```python
from build123d import *

# Parameters (mm, degrees)
SKETCH1_W           = 6.35
SKETCH1_H           = 20.32
SKETCH1_R           = 2.032
BOSS_EXTRUDE1_DEPTH = 11.43
SKETCH1_3_R         = 2.032
CUT_EXTRUDE1_DEPTH  = 6.35
SKETCH2_R           = 2.032
CUT_EXTRUDE2_DEPTH  = 17.558774109
CHAMFER1_SIZE       = 6.35
FILLET1_R           = 6.35
FILLET2_R           = 6.35
CHAMFER2_SIZE       = 0.635
CHAMFER3_SIZE       = 0.635


with BuildPart() as part:
    # Sketch1 → Boss-Extrude1 (new body)
    # profile 1 of 3: a face of its own
    with BuildSketch(Plane(origin=(0, 0, 0), x_dir=(1, 0, 0), z_dir=(0, 1, 0))):
        Rectangle(SKETCH1_W, SKETCH1_H)
        with Locations((0, -6.35)):
            Circle(SKETCH1_R, mode=Mode.SUBTRACT)
        with Locations((0, 6.35)):
            Circle(SKETCH1_R, mode=Mode.SUBTRACT)
    # profile 2 of 3: a face of its own
    with BuildSketch(Plane(origin=(0, 0, 0), x_dir=(1, 0, 0), z_dir=(0, 1, 0))):
        with Locations((0, -6.35)):
            Circle(SKETCH1_R)
    # profile 3 of 3: a face of its own
    with BuildSketch(Plane(origin=(0, 0, 0), x_dir=(1, 0, 0), z_dir=(0, 1, 0))):
        with Locations((0, 6.35)):
            Circle(SKETCH1_R)
    extrude(amount=BOSS_EXTRUDE1_DEPTH)

    # Sketch1<3> → Cut-Extrude1 (cut)
    with BuildSketch(Plane(origin=(0, 0, 0), x_dir=(1, 0, 0), z_dir=(0, 1, 0))):
        with Locations(Location((0, 6.35, 0), (0, 0, 270))):
            Circle(SKETCH1_3_R)
        with Locations(Location((0, -6.35, 0), (0, 0, 270))):
            Circle(SKETCH1_3_R)
    extrude(amount=CUT_EXTRUDE1_DEPTH, mode=Mode.SUBTRACT)

    # Sketch2 → Cut-Extrude2 (cut, through all)
    with BuildSketch(Plane(origin=(3.175, 0, 0), x_dir=(0, 0, -1), z_dir=(1, 0, 0))):
        with Locations((0, 7.62)):
            Circle(SKETCH2_R)
    extrude(amount=-CUT_EXTRUDE2_DEPTH, mode=Mode.SUBTRACT)

    # Chamfer1
    chamfer1_edges = [part.edges().sort_by_distance(p)[0] for p in [
        (0, 11.43, -10.16),
        (0, 11.43, 10.16),
    ]]
    chamfer(chamfer1_edges, length=CHAMFER1_SIZE)

    # Fillet1
    fillet1_edges = [part.edges().sort_by_distance(p)[0] for p in [
        (0, 11.43, 3.81),
        (0, 11.43, -3.81),
    ]]
    fillet(fillet1_edges, radius=FILLET1_R)

    # Fillet2
    fillet2_edges = [part.edges().sort_by_distance(p)[0] for p in [
        (0, 5.08, -10.16),
        (0, 5.08, 10.16),
    ]]
    fillet(fillet2_edges, radius=FILLET2_R)

    # Chamfer2
    chamfer2_edges = [part.edges().sort_by_distance(p)[0] for p in [
        (3.175, 11.43, 0),
        (-3.175, 11.43, 0),
        (-3.175, 8.255, -6.985),
        (-3.175, 10.946635031, 3.609783674),
        (-3.175, 10.946635031, -3.609783674),
        (3.175, 8.255, 6.985),
        (3.175, 10.946635031, 3.609783674),
        (3.175, 10.946635031, -3.609783674),
        (-3.175, 0, 0),
        (-3.175, 1.224871939, -10.16),
        (3.175, 1.224871939, -10.16),
        (3.175, 8.255, -6.985),
        (3.175, 1.224871939, 10.16),
        (3.175, 4.879783674, 9.676635031),
        (3.175, 4.879783674, -9.676635031),
        (-3.175, 1.224871939, 10.16),
        (0, 0, -10.16),
        (-3.175, 8.255, 6.985),
        (-3.175, 4.879783674, 9.676635031),
        (-3.175, 4.879783674, -9.676635031),
        (3.175, 0, 0),
        (0, 0, 10.16),
    ]]
    chamfer(chamfer2_edges, length=CHAMFER2_SIZE)

    # Chamfer3
    # the kernel refuses this chamfer: 0.635 mm, written as the material it takes off along each edge
    with BuildSketch(Plane(origin=(0, 0, 6.35), x_dir=(0, 0, 1), z_dir=(-1, 0, 0))) as chamfer3_piece_1:
        Polygon((2.032 + CHAMFER3_SIZE, 0), (2.032, CHAMFER3_SIZE), (2.032, 0), align=None)
    revolve(axis=Axis((0, 0, 6.35), (0, 1, 0)), mode=Mode.SUBTRACT)
    with BuildSketch(Plane(origin=(0, 0, -6.35), x_dir=(0, 0, 1), z_dir=(-1, 0, 0))) as chamfer3_piece_2:
        Polygon((2.032 + CHAMFER3_SIZE, 0), (2.032, CHAMFER3_SIZE), (2.032, 0), align=None)
    revolve(axis=Axis((0, 0, -6.35), (0, 1, 0)), mode=Mode.SUBTRACT)
    with BuildSketch(Plane(origin=(-3.175, 7.62, 0), x_dir=(0, 0, -1), z_dir=(0, -1, 0))) as chamfer3_piece_3:
        Polygon((2.032 + CHAMFER3_SIZE, 0), (2.032, CHAMFER3_SIZE), (2.032, 0), align=None)
    revolve(axis=Axis((-3.175, 7.62, 0), (1, 0, 0)), mode=Mode.SUBTRACT)
    with BuildSketch(Plane(origin=(3.175, 7.62, 0), x_dir=(0, 0, -1), z_dir=(0, -1, 0))) as chamfer3_piece_4:
        Polygon((2.032, -CHAMFER3_SIZE), (2.032 + CHAMFER3_SIZE, 0), (2.032, 0), align=None)
    revolve(axis=Axis((3.175, 7.62, 0), (1, 0, 0)), mode=Mode.SUBTRACT)


solid = part.part
```
Check sheet for the modelled part. Datum: model origin and axes. Units: mm. A direction names the side the tool comes from. Give positions to 0.01 mm unless a question says otherwise; leave off trailing zeros. Write each loop counter-clockwise with the first axis right and the second up, starting at its lowest first coordinate (ties: lowest second). Pieces come first, ordered by that corner, then holes. Notation, with made-up numbers: (18, -21) -> (46, -21) arc R38 ccw to (46, 17) -> close; hole circle Ø4 at (-34, 12.5). An arc over 180 degrees is marked (long way). Use CSV: the item, a comma, the result in double quotes. Start each with the question number.
Q1. Cross-section at D-D on y = 7.62. Enter the section's corners in (x, z) (3 decimals).
Q2. Cross-section at C-C on x = 0. Enter the section's corners in (y, z) (3 decimals).
Q3. Release check for a two-part mould opening along X. For faces 1 (the flat face through (-2.85, 8.02, 6.78)), 2 (the flat face through (0, 6.35, -6)), 3 (the flat face through (-0.04, 8.27, -6.97)) record: +X half, -X half, draft (parallel to the pull), parting line (faces both ways), or undercut.
Q4. Scan lines: line 1 along X through (y, z) = (4.1, -6.35) (3 decimals); line 2 along Y through (x, z) = (-0.6, 0); line 3 along Z through (x, y) = (-0.75, 4.5). Record each from-to range of solid material in increasing order.
Q5. Cross-section at B-B on y = 2. Enter the section's corners in (x, z) (3 decimals), and give its area (3 significant figures).
Q6. Cross-section at A-A on z = 0. Enter the section's corners in (x, y) (3 decimals).
Q7. Depth check by flat-ended pin: P1, Ø1.5, axis at x = 2.5, y = 7.5, coming from the -Z side; P2, Ø3.5, axis at x = 0, z = -6.35, coming from the -Y side; P3, Ø1, axis at x = 1.5, z = 5, coming from the +Y side. Enter the tip coordinate at first touch or a pass-through.
Q8. Tool access check on faces 4 (the flat face through (0, 6.35, 6)), 5 (the flat face through (-2.85, 8.05, -6.75)). Record the directions out of +Z, -Z, +X, -X, +Y, -Y that give a thin tool (end or side, any length) a straight path to the whole face; none if there is none.
Working result:
1,outline,"(-3.175, -6.722) -> (-2.54, -7.62) -> (2.54, -7.62) -> (3.175, -6.722) -> (3.175, -2.667) -> (2.54, -2.032) -> (-2.54, -2.032) -> (-3.175, -2.667) -> close; (-3.175, 2.667) -> (-2.54, 2.032) -> (2.54, 2.032) -> (3.175, 2.667) -> (3.175, 6.722) -> (2.54, 7.62) -> (-2.54, 7.62) -> (-3.175, 6.722) -> close"
2,outline,"(0, -9.525) -> (0.635, -10.16) -> (2.45, -10.16) arc R6.35 ccw to (6.94, -8.3) -> (9.57, -5.67) arc R6.35 ccw to (11.43, -1.18) -> (11.43, 1.18) arc R6.35 ccw to (9.57, 5.67) -> (6.94, 8.3) arc R6.35 ccw to (2.45, 10.16) -> (0.635, 10.16) -> (0, 9.525) -> (0, 9.017) -> (0.635, 8.382) -> (6.35, 8.382) -> (6.35, 4.318) -> (0.635, 4.318) -> (0, 3.683) -> (0, -3.683) -> (0.635, -4.318) -> (6.35, -4.318) -> (6.35, -8.382) -> (0.635, -8.382) -> (0, -9.017) -> close; hole circle Ø4.064 at (7.62, 0)"
3,face 1,"-X half"
3,face 2,"undercut"
3,face 3,"draft"
4,line 1,"x = -3.175 to -2.032, 2.032 to 3.175"
4,line 2,"y = 0 to 5.59, 9.65 to 11.43"
4,line 3,"z = -9.82 to -8.24, -4.46 to 4.46, 8.24 to 9.82"
5,outline,"(-3.175, -9.525) -> (-2.54, -10.16) -> (2.54, -10.16) -> (3.175, -9.525) -> (3.175, 9.525) -> (2.54, 10.16) -> (-2.54, 10.16) -> (-3.175, 9.525) -> close; hole circle Ø4.064 at (0, -6.35); hole circle Ø4.064 at (0, 6.35)"
5,area,"102 mm^2"
6,outline,"(-3.175, 0.635) -> (-2.54, 0) -> (2.54, 0) -> (3.175, 0.635) -> (3.175, 4.953) -> (2.54, 5.588) -> (-2.54, 5.588) -> (-3.175, 4.953) -> close; (-3.175, 10.287) -> (-2.54, 9.652) -> (2.54, 9.652) -> (3.175, 10.287) -> (3.175, 10.795) -> (2.54, 11.43) -> (-2.54, 11.43) -> (-3.175, 10.795) -> close"
7,P1,"stops at z = -8.48"
7,P2,"stops at y = 6.35"
7,P3,"stops at y = 10.49"
8,face 4,"-Y"
8,face 5,"-Z, -X, +Y"
